Verification items for this drawing (mm, ordinates from the low corner). A direction names the side the tool comes from. Give positions to 0.01 mm unless a question says otherwise; leave off trailing zeros. Write each loop counter-clockwise with the first axis right and the second up, starting at its lowest first coordinate (ties: lowest second). Pieces come first, ordered by that corner, then holes. Notation, with made-up numbers: M -33.5,-21 L -14.5,-21 A16 ccw -14.5,-9 Z; hole C -8,31 d1. An arc over 180 degrees is marked long. Use one line per item in the form item = value. Start each with the question number.
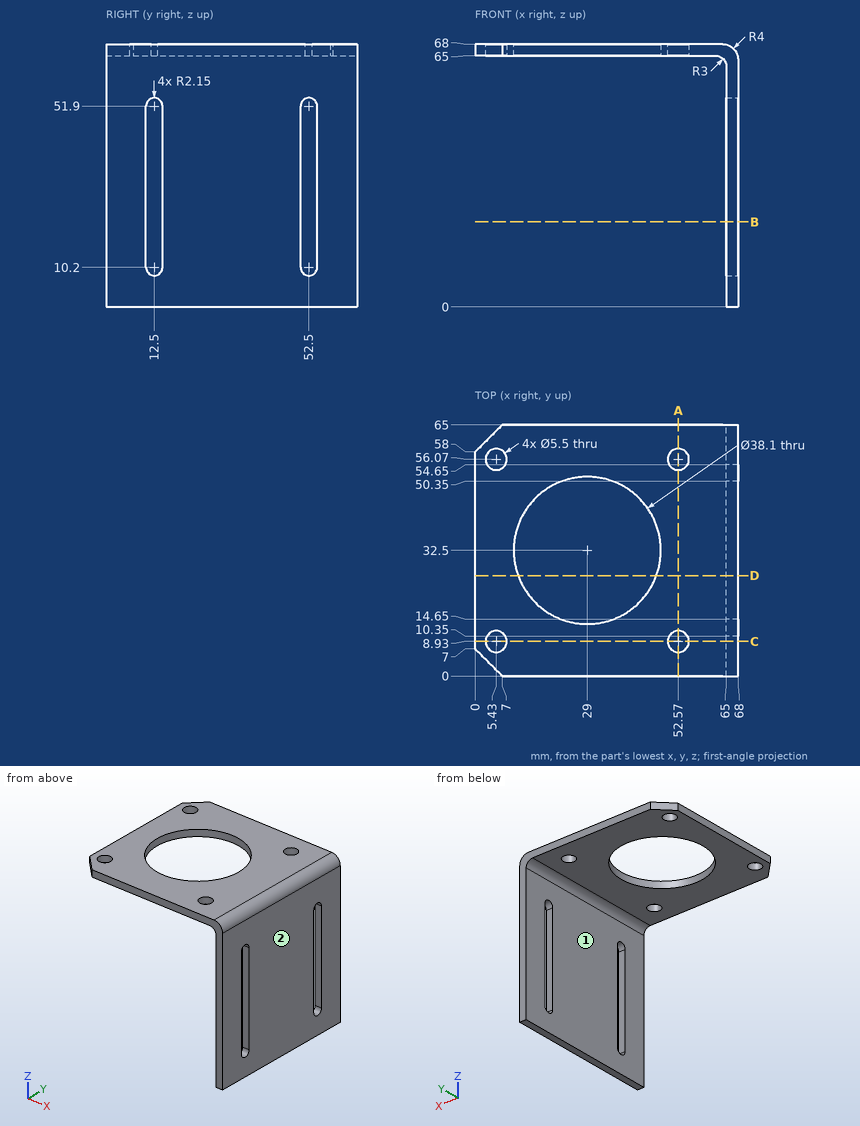
(1) Thickness scan on probe 1 along Y at (x, z) = (52.57, 67.2); probe 2 along X at (y, z) = (56, 66); probe 3 along Y at (x, z) = (52, 66). Record the ranges inside material, lowest first. Write a range as [from, to].
(2) Sectioned sample at D-D, the plane y = 26. Record the boundary of the cut face in (x, z), plus the area to 3 significant figures.
(3) Sectioned sample at B-B, the plane z = 22. Record the boundary of the cut face in (x, y).
(4) Sectioned sample at A-A, the plane x = 52.57. Record the boundary of the cut face in (y, z).
(5) Depth check by flat-ended pin: pin 1 (3.5 mm diameter, centred on x = 5.43, y = 8.93, fed in from +Z); pin 2 (6.5 mm diameter, centred on x = 5.43, y = 56.07, fed in from +Z); pin 3 (4 mm diameter, centred on y = 30, z = 42, fed in from -X). Enter the tip coordinate at first touch or a pass-through.
(6) Sectioned sample at C-C, the plane y = 8.93. Record the boundary of the cut face in (x, z), plus the area to 3 significant figures.
(7) Tool access check on the marked faces 1 and 2. Record the directions out of +Z, -Z, +X, -X, +Y, -Y that give a thin tool (end or side, any length) a straight path to the whole face; none if there is none.
Numbers:
q1.probe_1 = [0, 6.18], [11.68, 53.32], [58.82, 65]
q1.probe_2 = [0, 2.68], [8.18, 49.82], [55.32, 67.46]
q1.probe_3 = [0, 6.24], [11.62, 53.38], [58.76, 65]
q2.outline = M 0,65 L 11.09,65 L 11.09,68 L 0,68 Z; M 46.91,65 L 62,65 A3 cw 65,62 L 65,0 L 68,0 L 68,64 A4 ccw 64,68 L 46.91,68 Z
q2.area = 290 mm2
q3.outline = M 65,0 L 68,0 L 68,10.35 L 65,10.35 Z; M 65,14.65 L 68,14.65 L 68,50.35 L 65,50.35 Z; M 65,54.65 L 68,54.65 L 68,65 L 65,65 Z
q4.outline = M 0,65 L 6.18,65 L 6.18,68 L 0,68 Z; M 11.68,65 L 53.32,65 L 53.32,68 L 11.68,68 Z; M 58.82,65 L 65,65 L 65,68 L 58.82,68 Z
q5.pin_1 = through
q5.pin_2 = 68
q5.pin_3 = 65
q6.outline = M 0,65 L 2.68,65 L 2.68,68 L 0,68 Z; M 8.18,65 L 49.82,65 L 49.82,68 L 8.18,68 Z; M 55.32,65 L 62,65 A3 cw 65,62 L 65,0 L 68,0 L 68,64 A4 ccw 64,68 L 55.32,68 Z
q6.area = 364 mm2
q7.face_1 = -Z, -X, +Y, -Y
q7.face_2 = +Z, -Z, +X, +Y, -Y
